Build history of the part. All positions in model axes, mm. Give positions to 0.01 mm unless a question says otherwise; leave off trailing zeros. Write each loop counter-clockwise with the first axis right and the second up, starting at its lowest first coordinate (ties: lowest second). Pieces come first, ordered by that corner, then holes. Notation, with made-up numbers: (83, -13.75) -> (141, -13.75) arc R10 ccw to (141, -3.75) -> close; hole circle Ø3 at (-31.5, 68). An arc over 180 degrees is marked (long way). Put each result on its own line as item: value. Start each with the question number.
Item 1: Slice it at C-C, the plane x = -14. List the corners of the cut face in (y, z) (3 decimals), plus the area to 3 significant figures.
Item 2: Slice it at A-A, the plane y = -6. List the corners of the cut face in (x, z) (3 decimals), plus the area to 3 significant figures.
Item 3: Flat gauge pins, fed straight in: pin 1 Ø2.5 at (x, z) = (-43.5, 2) entering from +Y; pin 2 Ø0.5 at (x, y) = (64, -0.5) entering from +Z (3 decimals); pin 3 Ø1.2 at (x, z) = (2.5, 1) entering from -Y. Where does each tip first touch, or does it go through?
Item 4: Slice it at D-D, the plane x = 22. List the corners of the cut face in (y, z) (3 decimals).
Item 5: Drill centre lines: line 1 along X through (y, z) = (9, -0.35); line 2 along X through (y, z) = (3, 2.85); line 3 along Y through (x, z) = (59.5, 0.25). Where is each one in solid material? Low to high.
Item 6: Slice it at B-B, the plane z = -0.75. List the corners of the cut face in (x, y) (1 decimal), plus the area to 3 significant figures.
Autodesk Inventor part; units mm, degrees
ref_plane "YZ Plane" through (0, 0, 0) normal (1, 0, 0) x (0, 1, 0)
ref_plane "XZ Plane" through (0, 0, 0) normal (0, 1, 0) x (-1, 0, 0)
ref_plane "XY Plane" through (0, 0, 0) normal (0, 0, 1) x (1, 0, 0)
sketch "Skizze1" plane through (0, 0, 0) normal (0, 0, 1) x (1, 0, 0)
  line L0 (-68.016, 1.808) -> (67.584, 1.808)
  line L1 (67.584, 1.808) -> (67.584, -2.192)
  line L2 (67.584, -2.192) -> (-68.016, -2.192)
  line L3 (-68.016, -2.192) -> (-68.016, 1.808)
  line L4 (-68.016, 1.808) -> (67.584, -2.192) construction
  line L5 (67.584, 1.808) -> (-68.016, -2.192) construction
  point P0 (0, 0)
  point P1 (-0.216, -0.192)
  point P2 (-0.216, -0.192)
  dimension "d0" = 135.6
  dimension "d1" = 4
extrude "Extrusion1" add sketch "Skizze1" along normal mid plane 3.25
ref_plane "Arbeitsebene1" through (-68.016, -0.192, 1.625) normal (0, -1, 0) x (1, 0, 0)
sketch "Skizze2" plane through (-68.016, -0.192, 1.625) normal (0, -1, 0) x (1, 0, 0)
  line L0 (0, -3.25) -> (0, 0)
  line L1 (0, -3.25) -> (135.6, -3.25)
  line L2 (0, 0) -> (2.85, 0)
  line L3 (2.85, 0) -> (2.85, -3.25)
  line L4 (2.85, -3.25) -> (0, -3.25)
  line L5 (0, -3.25) -> (0, 0)
  line L6 (0, 0) -> (0, 1.75)
  line L7 (0, 1.75) -> (2.85, 0)
  line L8 (135.6, -3.25) -> (135.6, 0)
  line L9 (135.6, 0) -> (132.75, 0)
  line L10 (132.75, 0) -> (132.75, -3.25)
  line L11 (132.75, -3.25) -> (135.6, -3.25)
  line L12 (135.6, -3.25) -> (135.6, 0)
  line L13 (135.6, 0) -> (135.6, 1.75)
  line L14 (135.6, 1.75) -> (132.75, 0)
  point P0 (68.016, -1.625)
  dimension "d4" = 2.85
  dimension "d5" = 1.75
  dimension "d6" = 2.85
extrude "Extrusion2" add sketch "Skizze2" along normal mid plane 19.7
sketch "Skizze3" plane through (0, 0, 1.625) normal (0, 0, 1) x (1, 0, 0)
  circle A0 centre (0, 0) radius 3.8975
  dimension "d9" = 7.795
extrude "Extrusion3" cut sketch "Skizze3" against normal through all
sketch "Skizze4" plane through (0, 0, -1.625) normal (0, 0, -1) x (-1, 0, 0)
  line L0 (0.0769, -0.1614) -> (6.2269, -0.1614) construction
  circle A0 centre (0.0001, -0.1921) radius 2.495
  circle A1 centre (0.0001, -0.1921) radius 5.295
  line L1 (-24.5999, -1.5921) -> (24.6001, -1.5921)
  point P0 (-5.2949, -0.1921)
  point P1 (5.2951, -0.1921)
  point P2 (2.0653, -1.5921)
  point P3 (5.1066, -1.5921)
  point P4 (-5.1065, -1.5921)
  point P5 (-2.0651, -1.5921)
  dimension "d27" = 2.8
  dimension "d28" = 4.99
  dimension "d29" = 1.4
extrude "Extrusion4" add sketch "Skizze4" against normal blind 5.5 contours A0 L1 A1 picked at (4.3097, 0.2335)
sketch "Skizze5" plane through (0, 0, 1.625) normal (0, 0, 1) x (1, 0, 0)
  line L0 (-4.9028, 1.808) -> (-65.166, 1.808)
  line L1 (-3.2227, -2.192) -> (-65.166, -2.192)
  line L2 (-3.2094, 1.808) -> (-63.2094, 1.808)
  line L3 (-63.2094, 1.808) -> (-63.2094, -2.192)
  line L4 (-63.2094, -2.192) -> (-3.2094, -2.192)
  line L5 (-3.2094, -2.192) -> (-3.2094, 1.808)
  line L6 (3.2227, -2.192) -> (64.734, -2.192)
  line L7 (3.1164, 1.808) -> (63.1164, 1.808)
  line L8 (63.1164, 1.808) -> (63.1164, -2.192)
  line L9 (63.1164, -2.192) -> (3.1164, -2.192)
  line L10 (3.1164, -2.192) -> (3.1164, 1.808)
  point P0 (0, 0)
  point P1 (-8.6889, 1.808)
  point P2 (-8.6001, -2.192)
  point P3 (8.6889, 1.808)
  point P4 (8.6001, -2.192)
  point P5 (3.1164, -2.192)
  point P6 (-3.2094, -2.192)
  point P7 (-63.2094, 1.808)
  point P8 (63.1164, -2.192)
  point P9 (-2.0688, 1.808)
  dimension "d17" = 60
  dimension "d18" = 60
extrude "Extrusion5" add sketch "Skizze5" along normal blind 2.25
sketch "Skizze6" plane through (-65.166, -2.192, -1.625) normal (0, -1, 0) x (1, 0, 0)
  line L0 (1.9566, 5.5) -> (61.9566, 5.5)
  line L1 (1.9566, 5.5) -> (61.9566, 5.5)
  line L2 (56.9566, 5.5) -> (56.9566, 3.25)
  line L3 (56.9566, 3.25) -> (1.9566, 3.25)
  line L4 (1.9566, 3.25) -> (1.9566, 5.5)
  line L5 (61.9566, 5.5) -> (1.9566, 3.25)
  line L6 (128.2824, 3.25) -> (128.2824, 5.5)
  line L7 (128.2824, 5.5) -> (73.2824, 5.5)
  line L8 (73.2824, 5.5) -> (73.2824, 3.25)
  line L9 (73.2824, 3.25) -> (128.2824, 3.25)
  line L10 (128.2824, 3.25) -> (128.2824, 5.5)
  line L11 (73.2824, 5.5) -> (128.2824, 3.25)
  point P0 (65.166, 1.625)
  point P1 (56.5659, 5.5)
  point P2 (56.5659, 5.5)
  point P3 (56.5659, 5.5)
  dimension "d21" = 55
  dimension "d22" = 2.25
  dimension "d23" = 55
  dimension "d26" = 2.25
extrude "Extrusion6" cut sketch "Skizze6" against normal through all contours L0 L2 L5 L4 | L0 L5 L2 | L11 L7 L6
properties part number "2024_08_23_Holder_NMR_tube"
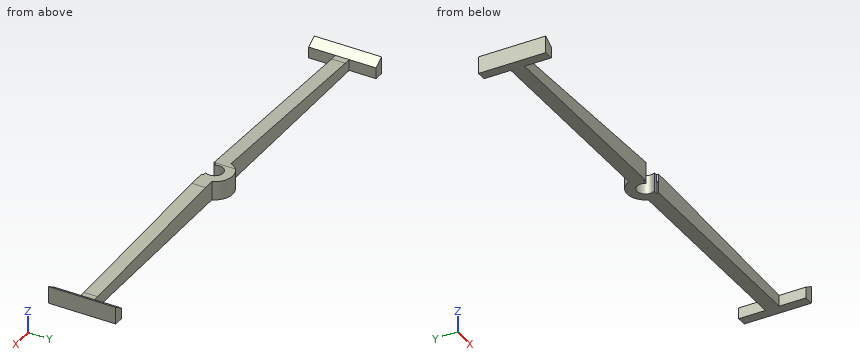
Values follow:
1. outline: (-2.192, -1.625) -> (1.808, -1.625) -> (1.808, 3.47) -> (-2.192, 3.47) -> close
1. area: 20.4 mm2
2. outline: (-68.016, -1.625) -> (-65.166, -1.625) -> (-65.166, 1.625) -> (-68.016, 3.375) -> close; (64.734, -1.625) -> (67.584, -1.625) -> (67.584, 3.375) -> (64.734, 1.625) -> close
2. area: 23.5 mm2
3. pin 1: y = 1.81
3. pin 2: z = 1.625
3. pin 3: y = -1.59
4. outline: (-2.192, -1.625) -> (1.808, -1.625) -> (1.808, 3.307) -> (-2.192, 3.307) -> close
5. line 1: -68.02 to -65.17, 64.73 to 67.58
5. line 2: -68.02 to -67.16, -4.22 to 4.22, 66.73 to 67.58
5. line 3: -2.19 to 1.81
6. outline: (-68, -10) -> (-65.2, -10) -> (-65.2, -2.2) -> (-3.2, -2.2) arc R3.9 cw to (-3.6, -1.6) -> (-2.1, -1.6) arc R2.5 cw (long way) to (2.1, -1.6) -> (3.6, -1.6) arc R3.9 cw to (3.2, -2.2) -> (64.7, -2.2) -> (64.7, -10) -> (67.6, -10) -> (67.6, 9.7) -> (64.7, 9.7) -> (64.7, 1.8) -> (4.9, 1.8) arc R5.3 ccw to (-4.9, 1.8) -> (-65.2, 1.8) -> (-65.2, 9.7) -> (-68, 9.7) -> close
6. area: 635 mm2
